For this review, take the finished solid that the model builds, in its own axes (mm). Give positions to 0.01 mm unless a question says otherwise; leave off trailing zeros. Order: outer loops, then holes, each group sorted by start corner. A loop starts at its lowest first (then second) coordinate and runs counter-clockwise, first axis right, second up. Notation, with made-up numbers: M -15,26 L 41,26 A19 cw 41,55 Z; hole C 79.5,-19.75 d1. An arc over 180 degrees is marked long. Answer as CSV lines item,"result". Start each with the question number.
1. We need section B-B, the plane z = 86.5. Give the boundary of the cut face in (x, y), and give its area (3 significant figures).
2. We need section C-C, the plane x = 20. Give the boundary of the cut face in (y, z).
3. Clearance check with flat-ended pins moving along their axes: P1, Ø0.6, axis at x = 85, y = 1, coming from the +Z side; P2, Ø1.5, axis at x = 74.5, y = 8, coming from the -Z side; P3, Ø7, axis at x = 170.5, z = 53.5, coming from the +Y side. State where each tip first meets the part, or that it passes through.
4. For line 1 along Z through (x, y) = (173.5, 4.1); line 2 along Z through (x, y) = (20, 3.05); line 3 along X through (y, z) = (6.6, 48), list the stretches that pass through material, from the lowest coordinate up.
5. We need section A-A, the plane x = 138. Give the boundary of the cut face in (y, z).
Autodesk Inventor part; units mm, degrees
ref_plane "YZ Plane" through (0, 0, 0) normal (1, 0, 0) x (0, 1, 0)
ref_plane "XZ Plane" through (0, 0, 0) normal (0, 1, 0) x (-1, 0, 0)
ref_plane "XY Plane" through (0, 0, 0) normal (0, 0, 1) x (1, 0, 0)
sketch "스케치1" plane through (0, 0, 0) normal (0, 1, 0) x (-1, 0, 0)
  line L0 (0, 0) -> (-206, 0)
  line L1 (-210, 4) -> (-210, 190)
  line L2 (-206, 194) -> (0, 194)
  line L3 (0, 194) -> (0, 0)
  line L4 (-40, 0) -> (-40, 194)
  line L5 (-20, 0) -> (-20, 194)
  circle A0 centre (-20, 97) radius 3.5
  circle A1 centre (-20, 48) radius 3.5
  circle A2 centre (-20, 146) radius 3.5
  arc A3 (-210, 4) -> (-206, 0) centre (-206, 4) ccw
  arc A4 (-206, 194) -> (-210, 190) centre (-206, 190) ccw
  circle A5 centre (-20, 97) radius 2.25
  circle A6 centre (-20, 146) radius 2.25
  circle A7 centre (-20, 48) radius 2.25
  line L6 (-40, 194) -> (-96.2917, 161.5)
  line L7 (-40, 194) -> (25, 194) construction
  line L8 (-96.2917, 161.5) -> (-166.2917, 161.5)
  line L9 (-166.2917, 161.5) -> (-189.6101, 194)
  line L10 (-210, 161.5) -> (-200, 144.1795)
  line L11 (-210, 161.5) -> (-190, 161.5) construction
  line L12 (-210, 97) -> (-40, 97)
  line L13 (-40, 0) -> (-96.2917, 32.5)
  line L14 (-96.2917, 32.5) -> (-166.2917, 32.5)
  line L15 (-166.2917, 32.5) -> (-189.6101, 0)
  line L16 (-210, 32.5) -> (-200, 49.8205)
  line L17 (-200, 144.1795) -> (-200, 49.8205)
  line L18 (-166.2917, 32.5) -> (-200, 32.5)
  line L19 (-200, 32.5) -> (-200, 49.8205)
  line L20 (-200, 144.1795) -> (-200, 161.5)
  line L21 (-166.2917, 161.5) -> (-200, 161.5)
  point P0 (-210, 194)
  point P1 (-210, 0)
  dimension "d0" = 210
  dimension "d1" = 194
  dimension "d2" = 40
  dimension "d3" = 20
  dimension "d4" = 7
  dimension "d5" = 7
  dimension "d6" = 7
  dimension "d7" = 49
  dimension "d8" = 49
  dimension "d9" = 4
  dimension "d17" = 4.5
  dimension "d18" = 4.5
  dimension "d19" = 4.5
  dimension "d82" = 65
  dimension "d83" = 150
  dimension "d84" = 70
  dimension "d85" = 40
  dimension "d86" = 20
  dimension "d87" = 60
extrude "돌출1" add sketch "스케치1" along normal blind 10
extrude "돌출2" cut sketch "스케치1" along normal blind 3 contours A1 L5 A7 | L5 A7 A1 | A7 L5 | L5 A7 | A2 L5 A6 | L5 A6 A2 | A0 L5 A5 | L5 A5 A0 | A6 L5 | L5 A6 | A5 L5 | L5 A5
sketch "스케치2" plane through (0, 0, 0) normal (0, -1, 0) x (1, 0, 0)
  line L0 (176, 45) -> (83, 45)
  line L1 (79, 49) -> (79, 142)
  line L2 (83, 146) -> (176, 146)
  line L3 (180, 142) -> (180, 49)
  line L4 (206, 0) -> (0, 0)
  line L5 (210, 190) -> (210, 4)
  arc A0 (176, 45) -> (180, 49) centre (176, 49) ccw
  arc A1 (180, 142) -> (176, 146) centre (176, 142) ccw
  arc A2 (83, 146) -> (79, 142) centre (83, 142) ccw
  arc A3 (79, 49) -> (83, 45) centre (83, 49) ccw
  line L6 (180, 45) -> (169.5, 45)
  line L7 (169.5, 45) -> (169.5, 55.5)
  line L8 (169.5, 55.5) -> (180, 55.5)
  line L9 (180, 55.5) -> (180, 45)
  line L10 (79, 45) -> (89.5, 45)
  line L11 (89.5, 45) -> (89.5, 55.5)
  line L12 (89.5, 55.5) -> (79, 55.5)
  line L13 (79, 55.5) -> (79, 45)
  line L14 (180, 146) -> (169.5, 146)
  line L15 (169.5, 146) -> (169.5, 135.5)
  line L16 (169.5, 135.5) -> (180, 135.5)
  line L17 (180, 135.5) -> (180, 146)
  line L18 (79, 146) -> (89.5, 146)
  line L19 (89.5, 146) -> (89.5, 135.5)
  line L20 (89.5, 135.5) -> (79, 135.5)
  line L21 (79, 135.5) -> (79, 146)
  circle A4 centre (173.5, 51.5) radius 1.6
  circle A5 centre (85.5, 51.5) radius 1.6
  circle A6 centre (85.5, 139.5) radius 1.6
  circle A7 centre (173.5, 139.5) radius 1.6
  line L22 (173.5, 51.5) -> (169.5, 51.5)
  line L23 (170.4978, 51.5) -> (171.9989, 54.1)
  line L24 (171.9989, 54.1) -> (175.0011, 54.1)
  line L25 (175.0011, 54.1) -> (176.5022, 51.5)
  line L26 (176.5022, 51.5) -> (175.0011, 48.9)
  line L27 (175.0011, 48.9) -> (171.9989, 48.9)
  line L28 (171.9989, 48.9) -> (170.4978, 51.5)
  line L29 (85.5, 51.5) -> (89.5, 51.5)
  line L30 (88.5022, 51.5) -> (87.0011, 48.9)
  line L31 (87.0011, 48.9) -> (83.9989, 48.9)
  line L32 (83.9989, 48.9) -> (82.4978, 51.5)
  line L33 (82.4978, 51.5) -> (83.9989, 54.1)
  line L34 (83.9989, 54.1) -> (87.0011, 54.1)
  line L35 (87.0011, 54.1) -> (88.5022, 51.5)
  line L36 (85.5, 139.5) -> (89.5, 139.5)
  line L37 (88.5022, 139.5) -> (87.0011, 136.9)
  line L38 (87.0011, 136.9) -> (83.9989, 136.9)
  line L39 (83.9989, 136.9) -> (82.4978, 139.5)
  line L40 (82.4978, 139.5) -> (83.9989, 142.1)
  line L41 (83.9989, 142.1) -> (87.0011, 142.1)
  line L42 (87.0011, 142.1) -> (88.5022, 139.5)
  line L43 (173.5, 139.5) -> (169.5, 139.5)
  line L44 (170.4978, 139.5) -> (171.9989, 142.1)
  line L45 (171.9989, 142.1) -> (175.0011, 142.1)
  line L46 (175.0011, 142.1) -> (176.5022, 139.5)
  line L47 (176.5022, 139.5) -> (175.0011, 136.9)
  line L48 (175.0011, 136.9) -> (171.9989, 136.9)
  line L49 (171.9989, 136.9) -> (170.4978, 139.5)
  point P0 (174.75, 55.5)
  dimension "d14" = 101
  dimension "d15" = 101
  dimension "d16" = 45
  dimension "d24" = 30
  dimension "d25" = 4
  dimension "d26" = 10.5
  dimension "d27" = 10.5
  dimension "d28" = 10.5
  dimension "d29" = 10.5
  dimension "d30" = 10.5
  dimension "d31" = 10.5
  dimension "d32" = 10.5
  dimension "d33" = 10.5
  dimension "d34" = 3.2
  dimension "d36" = 4
  dimension "d37" = 3.2
  dimension "d38" = 4
  dimension "d39" = 4
  dimension "d40" = 3.2
  dimension "d41" = 4
  dimension "d42" = 4
  dimension "d43" = 3.2
  dimension "d44" = 4
  dimension "d45" = 4
  dimension "d46" = 4
  dimension "d58" = 5.2
  dimension "d59" = 5.2
  dimension "d60" = 5.2
  dimension "d61" = 5.2
  dimension "d95" = 88
extrude "돌출3" cut sketch "스케치1" along normal blind 4 contours A1 L5 A7 | L5 A7 A1 | A7 L5 | L5 A7 | A2 L5 A6 | L5 A6 A2 | A0 L5 A5 | L5 A5 A0 | A6 L5 | L5 A6 | A5 L5 | L5 A5
extrude "돌출4" cut sketch "스케치1" along normal blind 10 contours A7 L5 | L5 A7 | A6 L5 | L5 A6 | A5 L5 | L5 A5
sketch "스케치4" plane through (0, 10, 0) normal (0, 1, 0) x (1, 0, 0)
  line L0 (176, -45) -> (83, -45)
  line L1 (180, -142) -> (180, -49)
  line L2 (79, -49) -> (79, -142)
  line L3 (83, -146) -> (176, -146)
  line L4 (79, -135.5) -> (79, -146)
  line L5 (79, -146) -> (89.5, -146)
  line L6 (180, -135.5) -> (180, -146)
  line L7 (180, -146) -> (169.5, -146)
  line L8 (180, -45) -> (169.5, -45)
  line L9 (180, -55.5) -> (180, -45)
  line L10 (79, -45) -> (89.5, -45)
  line L11 (79, -55.5) -> (79, -45)
  arc A0 (83, -45) -> (79, -49) centre (83, -49) ccw
  arc A1 (180, -49) -> (176, -45) centre (176, -49) ccw
  arc A2 (176, -146) -> (180, -142) centre (176, -142) ccw
  arc A3 (79, -142) -> (83, -146) centre (83, -142) ccw
  point P0 (0, 0)
extrude "돌출6" cut sketch "스케치4" against normal blind 3 contours A1 L1 A2 L3 A3 L2 A0 L0
extrude "돌출7" cut sketch "스케치2" against normal blind 10 contours A4 | A5 | A7 | A6
extrude "돌출8" cut sketch "스케치2" against normal blind 2 contours A4 | L23 L24 L25 L26 L27 L28 | A5 | L30 L31 L32 L33 L34 L35 | A7 | L44 L45 L46 L47 L48 L49 | A6 | L37 L38 L39 L40 L41 L42
sketch "스케치5" plane through (0, 7, 0) normal (0, 1, 0) x (1, 0, 0)
  line L0 (89.5, -55.5) -> (79, -55.5)
  line L1 (89.5, -45) -> (89.5, -55.5)
  line L2 (176, -45) -> (83, -45)
  line L3 (169.5, -45) -> (169.5, -55.5)
  line L4 (169.5, -55.5) -> (180, -55.5)
  line L5 (180, -142) -> (180, -49)
  line L6 (169.5, -135.5) -> (180, -135.5)
  line L7 (169.5, -146) -> (169.5, -135.5)
  line L8 (83, -146) -> (176, -146)
  line L9 (89.5, -146) -> (89.5, -135.5)
  line L10 (89.5, -135.5) -> (79, -135.5)
  line L11 (79, -49) -> (79, -142)
  point P0 (0, 0)
extrude "돌출9" cut sketch "스케치5" against normal blind 10
fillet "모깎기2" radius 3 12 edges at (169.5, 3.5, 55.5) (169.5, 3.5, 45) (180, 3.5, 55.5) (180, 3.5, 135.5) (169.5, 3.5, 135.5) (169.5, 3.5, 146) (89.5, 3.5, 146) (89.5, 3.5, 135.5) (79, 3.5, 135.5) (89.5, 3.5, 45) (79, 3.5, 55.5) (89.5, 3.5, 55.5)
extrude "돌출14" cut sketch "스케치1" along normal blind 10 contours L0 L15 L14 L13 | L6 L8 L9 L2
extrude "돌출15" cut sketch "스케치1" along normal blind 10 contours L17 L16 L1 L12 | L12 L1 L10 L17
extrude "돌출16" cut sketch "스케치1" along normal blind 10 contours L0 A3 L1 L16 L19 L18 L15 | L9 L21 L20 L10 L1 A4 L2
fillet "모깎기5" radius 3 9 edges at (200, 5, 32.5) (200, 5, 161.5) (148.1458, 10, 32.5) (200, 10, 97) (148.1458, 10, 161.5) (68.1458, 10, 16.25) (96.2917, 5, 32.5) (96.2917, 5, 161.5) (68.1458, 10, 177.75)
sketch "스케치11" plane through (0, 10, 0) normal (0, 1, 0) x (1, 0, 0)
  line L0 (34, 0) -> (94.0955, -34.6962)
  line L1 (34, 0) -> (0, 0)
  line L2 (0, 0) -> (0, -194)
  line L3 (0, -194) -> (34, -194)
  line L4 (94.0955, -159.3038) -> (34, -194)
  arc A0 (97.0955, -158.5) -> (94.0955, -159.3038) centre (97.0955, -164.5) ccw
  line L5 (197, -158.5) -> (97.0955, -158.5)
  line L6 (197, -35.5) -> (197, -158.5)
  line L7 (97.0955, -35.5) -> (197, -35.5)
  arc A1 (94.0955, -34.6962) -> (97.0955, -35.5) centre (97.0955, -29.5) ccw
  circle A2 centre (20, -48) radius 2.25
  circle A3 centre (20, -97) radius 2.25
  circle A4 centre (20, -146) radius 2.25
  arc A5 (176, -146) -> (180, -142) centre (176, -142) ccw
  line L8 (176, -146) -> (83, -146)
  arc A6 (79, -142) -> (83, -146) centre (83, -142) ccw
  line L9 (79, -142) -> (79, -49)
  arc A7 (83, -45) -> (79, -49) centre (83, -49) ccw
  line L10 (83, -45) -> (176, -45)
  arc A8 (180, -49) -> (176, -45) centre (176, -49) ccw
  line L11 (180, -49) -> (180, -142)
  line L12 (210, -97) -> (40, -97)
  arc A9 (54, -76) -> (56, -78) centre (56, -76) ccw
  line L13 (56, -78) -> (62, -78)
  arc A10 (62, -78) -> (64, -76) centre (62, -76) ccw
  line L14 (64, -76) -> (64, -60)
  arc A11 (64, -60) -> (62, -58) centre (62, -60) ccw
  line L15 (62, -58) -> (56, -58)
  arc A12 (56, -58) -> (54, -60) centre (56, -60) ccw
  line L16 (54, -60) -> (54, -76)
  line L17 (79, -58.5) -> (79, -132.5)
  line L18 (79, -73) -> (64, -73)
  line L19 (64, -73) -> (64, -63)
  line L20 (64, -63) -> (79, -63)
  line L21 (79, -63) -> (79, -73)
  dimension "d104" = 3
  dimension "d105" = 3
extrude "돌출19" cut sketch "스케치11" against normal blind 3 contours L18 L14 L20 L9
extrude "돌출20" cut sketch "스케치11" against normal blind 10 contours L14 A10 L13 A9 L16 A12 L15 A11
properties part number "XY_STAGE_BOARD1"
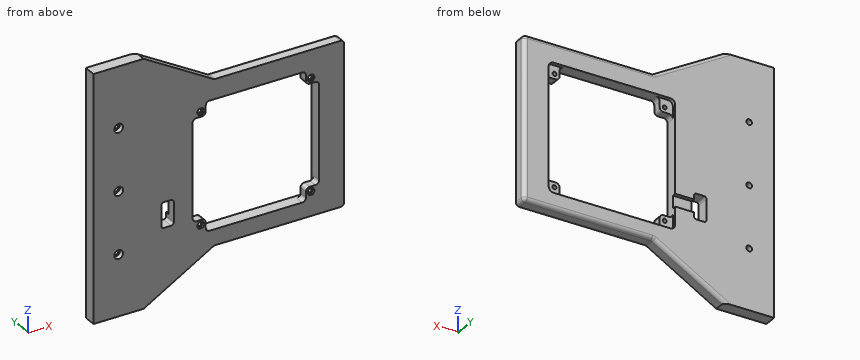
Result set:
1,outline,"M 0,0 L 79,0 L 79,10 L 0,10 Z; M 180,0 L 200,0 L 200,7 A3 ccw 197,10 L 180,10 Z"
1,area,"988 mm2"
2,outline,"M 0,0 L 10,0 L 10,45.75 L 4,45.75 L 4,44.5 L 0,44.5 Z; M 0,51.5 L 4,51.5 L 4,50.25 L 10,50.25 L 10,94.75 L 4,94.75 L 4,93.5 L 0,93.5 Z; M 0,100.5 L 4,100.5 L 4,99.25 L 10,99.25 L 10,143.75 L 4,143.75 L 4,142.5 L 0,142.5 Z; M 0,149.5 L 4,149.5 L 4,148.25 L 10,148.25 L 10,194 L 0,194 Z"
3,P1,"z = 168.19"
3,P2,"z = 19.62"
3,P3,"y = 7"
4,line 1,"32.5 to 49.9, 53.1 to 55.5, 135.5 to 137.9, 141.1 to 161.5"
4,line 2,"0 to 44.5, 51.5 to 93.5, 100.5 to 142.5, 149.5 to 194"
4,line 3,"0 to 17.75, 22.25 to 89.5, 169.5 to 200"
5,outline,"M 0,32.5 L 7,32.5 A3 ccw 10,35.5 L 10,45 L 0,45 Z; M 0,146 L 10,146 L 10,158.5 A3 ccw 7,161.5 L 0,161.5 Z"
